from build123d import *

# Parameters (mm, degrees)
SKETCH7_R                              = 55.5
BOSS_EXTRUDE1_DEPTH                    = 3
F_3_0MM_TRANSITIONAL_DOWEL_HOLE1_D     = 3
F_3_0MM_TRANSITIONAL_DOWEL_HOLE1_DEPTH = 25.4
F_3_0MM_TRANSITIONAL_DOWEL_HOLE1_TIP   = 0.901290929
F_4_0MM_DOWEL_HOLE1_D                  = 4
F_4_0MM_DOWEL_HOLE1_DEPTH              = 25.4
F_4_0MM_DOWEL_HOLE1_TIP                = 1.201721238


with BuildPart() as part:
    # Sketch7 → Boss-Extrude1 (new body)
    with BuildSketch(Plane(origin=(0, 0, 0), x_dir=(1, 0, 0), z_dir=(0, 1, 0))):
        with Locations(Location((0, 0, 0), (0, 0, 270))):
            Circle(SKETCH7_R)
    extrude(amount=BOSS_EXTRUDE1_DEPTH)

    # Ø3.0mm Transitional Dowel Hole1
    with Locations(Plane(origin=(0, 3, 0), x_dir=(1, 0, 0), z_dir=(0, 1, 0))):
        with Locations((-38.476262074, 27.999994228), (31.523738554, 19.999999725), (31.523741695, -20.000000275), (-38.476257677, -28.000005772)):
            Hole(F_3_0MM_TRANSITIONAL_DOWEL_HOLE1_D / 2, depth=F_3_0MM_TRANSITIONAL_DOWEL_HOLE1_DEPTH)
            with Locations((0, 0, -(F_3_0MM_TRANSITIONAL_DOWEL_HOLE1_DEPTH + F_3_0MM_TRANSITIONAL_DOWEL_HOLE1_TIP / 2))):  # 118° drill point
                Cone(0, F_3_0MM_TRANSITIONAL_DOWEL_HOLE1_D / 2, F_3_0MM_TRANSITIONAL_DOWEL_HOLE1_TIP, mode=Mode.SUBTRACT)

    # Ø4.0mm Dowel Hole1
    with Locations(Plane(origin=(0, 3, 0), x_dir=(1, 0, 0), z_dir=(0, 1, 0))):
        with Locations((-30.906824904, 32.5), (30.906824904, 32.5), (30.906824904, -32.5), (-30.906824904, -32.5)):
            Hole(F_4_0MM_DOWEL_HOLE1_D / 2, depth=F_4_0MM_DOWEL_HOLE1_DEPTH)
            with Locations((0, 0, -(F_4_0MM_DOWEL_HOLE1_DEPTH + F_4_0MM_DOWEL_HOLE1_TIP / 2))):  # 118° drill point
                Cone(0, F_4_0MM_DOWEL_HOLE1_D / 2, F_4_0MM_DOWEL_HOLE1_TIP, mode=Mode.SUBTRACT)


solid = part.part
Part model, mm, in its own coordinate system. Give positions to 0.01 mm unless a question says otherwise; leave off trailing zeros. Order: outer loops, then holes, each group sorted by start corner. A loop starts at its lowest first (then second) coordinate and runs counter-clockwise, first axis right, second up. Notation, with made-up numbers: (-31.75, 15) - (-1.75, 15) arc R21 ccw to (-1.75, 34) - close; hole circle Ø11 at (-35, -10). An arc over 180 degrees is marked (long way). Use a Markdown table: item, result.
1) Saw through at A-A on y = 2.25. Count the separate pieces of the cut face and the enclosed holes in it, plus the area to 3 significant figures.
Checked values:
| item | result |
|---|---|
| separate pieces | 1 |
| enclosed holes | 8 |
| area | 9,600 mm² |
2) Saw through at C-C on z = -20. List the corners of the cut face in (x, y).
Checked values:
| item | result |
|---|---|
| outline | (-51.77, 0) - (30.02, 0) - (30.02, 3) - (-51.77, 3) - close; (33.02, 0) - (51.77, 0) - (51.77, 3) - (33.02, 3) - close |
3) Probe L1, parallel to X at y = 2.2, z = -32.5; L2, parallel to Z at x = 31, y = 0.7; L3, parallel to Z at x = -33, y = 2.6. List the from-to ranges inside material, lowest first. Write a range as from..to.
Checked values:
| item | result |
|---|---|
| L1 | -44.99..-32.91, -28.91..28.91, 32.91..44.99 |
| L2 | -46.04..-34.5, -30.5..-21.41, -18.59..18.59, 21.41..30.5, 34.5..46.04 |
| L3 | -44.62..44.62 |
4) Two-plate mould, pull along X, no slides. Class faces 1 (the cylindrical face through (31.34, 1.479, -30.548)), 2 (the flat face through (1, 0, -1)), 3 (the cylindrical face through (31.34, 1.479, 34.452)), 4 (the cylindrical face through (46.798, 1.479, 29.836)): +X half, -X half, draft (parallel to the pull), parting line (faces both ways), or undercut.
Checked values:
| item | result |
|---|---|
| face 1 | undercut |
| face 2 | draft |
| face 3 | undercut |
| face 4 | parting line |
5) Saw through at B-B on z = -32.5. List the corners of the cut face in (x, y).
Checked values:
| item | result |
|---|---|
| outline | (-44.99, 0) - (-32.91, 0) - (-32.91, 3) - (-44.99, 3) - close; (-28.91, 0) - (28.91, 0) - (28.91, 3) - (-28.91, 3) - close; (32.91, 0) - (44.99, 0) - (44.99, 3) - (32.91, 3) - close |
6) Saw through at D-D on x = 22.5. List the corners of the cut face in (y, z), plus the area to 3 significant figures.
Checked values:
| item | result |
|---|---|
| outline | (0, -50.73) - (3, -50.73) - (3, 50.73) - (0, 50.73) - close |
| area | 304 mm² |
7) Flat gauge pin, fed straight in: P1, Ø1.5, axis at x = -14.5, y = 0.5, coming from the +Z side. Where does the tip first touch, or does it go through?
Checked values:
| item | result |
|---|---|
| P1 | z = 53.77 |
